```python
from build123d import *

# Parameters (mm, degrees)
SKETCH1_R                = 1.8
BOSS_EXTRUDE1_DEPTH      = 2
BOSS_EXTRUDE2_DEPTH      = 33
BOSS_EXTRUDE3_DEPTH      = 1
CHAMFER1_START           = 78.15897378
CHAMFER1_DEPTH           = 1.443375673
BOSS_EXTRUDE4_DEPTH      = 3
BOSS_EXTRUDE4_DEPTH_BACK = 0.0001
BOSS_EXTRUDE5_DEPTH      = 2.5
CUT_EXTRUDE1_DEPTH       = 3.0001


with BuildPart() as part:
    # Sketch1 → Boss-Extrude1 (new body)
    with BuildSketch(Plane(origin=(34.895003496, 0, 0), x_dir=(0, 0, -1), z_dir=(1, 0, 0))):
        with BuildLine():
            Line((-197.649446246, 296.929756404), (-189.949446246, 296.929756404))
            Line((-189.949446246, 296.929756404), (-189.949446246, 254.929756404))
            Line((-189.949446246, 254.929756404), (-196.543558796, 254.929756404))
            Line((-196.543558796, 254.929756404), (-231.255333696, 254.929756404))
            Line((-231.255333696, 254.929756404), (-234.649446246, 258.323868954))
            Line((-234.649446246, 258.323868954), (-234.649446246, 304.785643855))
            Line((-234.649446246, 304.785643855), (-231.255333696, 308.179756404))
            Line((-231.255333696, 308.179756404), (-227.755333696, 308.179756404))
            Line((-227.755333696, 308.179756404), (-224.361221147, 304.785643855))
            Line((-224.361221147, 304.785643855), (-220.634013353, 301.058436061))
            ThreePointArc((-220.634013353, 301.058436061), (-219.660743306, 300.408117807), (-218.512693009, 300.179756404))
            Line((-218.512693009, 300.179756404), (-213.899446246, 300.179756404))
            ThreePointArc((-213.899446246, 300.179756404), (-211.430377525, 299.74636844), (-209.256499056, 298.498018377))
            Line((-209.256499056, 298.498018377), (-208.488462922, 297.857611868))
            ThreePointArc((-208.488462922, 297.857611868), (-207.289081698, 297.168867005), (-205.926836886, 296.929756404))
            Line((-205.926836886, 296.929756404), (-197.649446246, 296.929756404))
        make_face()
        with Locations(Location((-198.399446246, 291.179756404, 0), (0, 0, 90))):
            Circle(SKETCH1_R, mode=Mode.SUBTRACT)
        with Locations(Location((-198.399446246, 260.179756404, 0), (0, 0, 90))):
            Circle(SKETCH1_R, mode=Mode.SUBTRACT)
        with Locations(Location((-229.399446246, 260.179756404, 0), (0, 0, 90))):
            Circle(SKETCH1_R, mode=Mode.SUBTRACT)
    extrude(amount=BOSS_EXTRUDE1_DEPTH)

    # Sketch2 → Boss-Extrude2 (add)
    with BuildSketch(Plane.ZY.offset(-34.895003496)):
        Polygon((192.949446246, 296.929756404), (192.949446246, 255.737509851), (192.949446246, 254.929756404), (189.949446246, 254.929756404), (189.949446246, 296.929756404), align=None)
    extrude(amount=BOSS_EXTRUDE2_DEPTH)

    # Sketch3 → Boss-Extrude3 (add)
    with BuildSketch(Plane(origin=(0, 296.929756404, 0), x_dir=(1, 0, 0), z_dir=(0, 1, 0))):
        Polygon((24.09465277, -192.949446246), (34.895003496, -196.599446246), (34.895003496, -192.949446246), align=None)
    extrude(amount=-BOSS_EXTRUDE3_DEPTH)

    # Chamfer1: read off the stored shape, not the designer's step
    # Chamfer1 outline → Chamfer1 (add)
    with BuildSketch(Plane(origin=(0, 0, 0), x_dir=(0.8164965809277265, -0.4082482904638619, 0.4082482904638633), z_dir=(0.5773502691896251, 0.5773502691896252, -0.5773502691896272)).offset(CHAMFER1_START)):
        Polygon((-15.59112598, -345.689799375), (-12.529263801, -347.457566328), (-12.529263801, -343.922032422), align=None)
    extrude(amount=CHAMFER1_DEPTH)

    # Sketch4 → Boss-Extrude4 (add, two sides: drawn at the far end of the back side and taken through both)
    with BuildSketch(Plane.XZ.offset(-254.929756404).offset(-BOSS_EXTRUDE4_DEPTH_BACK)):
        Polygon((1.895003496, 192.949446246), (34.895003496, 192.949446246), (34.895003496, 231.255333696), (36.895003496, 231.255333696), (36.895003496, 189.949446246), (1.895003496, 170.0501531), align=None)
    extrude(amount=BOSS_EXTRUDE4_DEPTH + BOSS_EXTRUDE4_DEPTH_BACK)

    # Sketch5 → Boss-Extrude5 (add)
    with BuildSketch(Plane.XZ.offset(-251.929756404)):
        Polygon((11.795887964, 192.949446246), (34.895003496, 212.102389971), (34.895003496, 192.949446246), align=None)
    extrude(amount=-BOSS_EXTRUDE5_DEPTH)

    # Sketch6 → Cut-Extrude1 (cut)
    with BuildSketch(Plane(origin=(0, 254.929856404, 0), x_dir=(1, 0, 0), z_dir=(0, 1, 0))):
        Polygon((1.895003496, -189.949446246), (36.895003496, -189.949446246), (1.895003496, -170.0501531), align=None)
    extrude(amount=-CUT_EXTRUDE1_DEPTH, mode=Mode.SUBTRACT)


solid = part.part
```
The model under review builds one solid part; all positions refer to its coordinate system, in mm. A direction names the side the tool comes from. Round coordinates to 2 decimals unless told otherwise and drop trailing zeros. Loops run counter-clockwise (first coordinate to the right, second up) from the corner with the lowest first, then second, coordinate; pieces in that order, holes last. Notation, with made-up numbers: (56.5, 65) - (78.5, 65) arc R16 ccw to (78.5, 77) - close; hole circle Ø3 at (73.25, 47). An arc over 180 degrees is marked (long way). Use a Markdown table: item, result. Add a question column.
Q1. Add section B-B (x = 33.5). State the section outline as (y, z) points.
Q2. Add section D-D (y = 288). State the section outline as (x, z) points (3 decimals), plus the area to 3 significant figures.
Q3. Add section C-C (z = 199.5). State the section outline as (x, y) points (3 decimals), plus the area to 3 significant figures.
Q4. For probe 1 along Z at (x, y) = (32, 257.5); probe 2 along X at (y, z) = (261, 225.5) (3 decimals); probe 3 along Y at (x, z) = (28, 195.5), list the stretches that pass through material, from the lowest coordinate up.
Q5. Insertion check: pin 1 Ø16.5 at (x, y) = (18.5, 280.5) entering from +Z; pin 2 Ø8 at (x, z) = (17, 198.5) entering from +Y; pin 3 Ø2 at (y, z) = (260.18, 229.4) entering from +X; pin 4 Ø10 at (x, z) = (31.5, 219) entering from +Y. Each pin has a flat end and moves straight along its axis. Give the tip position at first contact, or say it passes through.
Q6. Add section A-A (z = 230.5). State the section outline as (x, y) points (3 decimals).
Q7. Machinability: for faces 4 (the face through (18, 275, 192.949)), 5 (the face through (35.881, 258.853, 230.616)), 6 (the face through (29.42, 296.44, 194.75)), which of the approach directions +Z, -Z, +X, -X, +Y, -Y give a long, thin tool a straight path to every point of the face, cutting with its end or side? Answer none if there is none.
Q8. The part is to be moulded in two halves that separate along Z. For faces 1 (the face through (23, 296.93, 192)), 2 (the face through (35.881, 258.853, 199.616)), 3 (the face through (36, 253, 231.255)), say which applies: pulls with the +Z half, pulls with the -Z half, needs draft (parallel to the pull), parting line crosses it, or undercut.
Worked answers:
| question | item | result |
|---|---|---|
| 1 | outline | (251.93, 189.95) - (296.93, 189.95) - (296.93, 196.13) - (295.93, 196.13) - (295.93, 194.05) - (294.82, 192.95) - (254.43, 192.95) - (254.43, 210.95) - (251.93, 210.95) - close |
| 2 | outline | (1.895, 189.949) - (36.895, 189.949) - (36.895, 234.649) - (34.895, 234.649) - (34.895, 192.949) - (1.895, 192.949) - close |
| 2 | area | 188 mm² |
| 3 | outline | (19.696, 251.93) - (36.895, 251.93) - (36.895, 258.755) - (34.895, 258.755) - (34.895, 254.43) - (19.696, 254.43) - close; (34.895, 261.604) - (36.895, 261.604) - (36.895, 289.755) - (34.895, 289.755) - close; (34.895, 292.604) - (36.895, 292.604) - (36.895, 296.93) - (34.895, 296.93) - close |
| 3 | area | 117 mm² |
| 4 | probe 1 | 189.95 to 192.95 |
| 4 | probe 2 | 34.895 to 36.895 |
| 4 | probe 3 | 251.93 to 254.43 |
| 5 | pin 1 | z = 192.95 |
| 5 | pin 2 | y = 254.43 |
| 5 | pin 3 | through |
| 5 | pin 4 | y = 303.1 |
| 6 | outline | (34.895, 251.93) - (36.895, 251.93) - (36.895, 258.755) - (34.895, 258.755) - close; (34.895, 261.604) - (36.895, 261.604) - (36.895, 308.18) - (34.895, 308.18) - close |
| 7 | face 4 | +Z, -X |
| 7 | face 5 | +X, -X |
| 7 | face 6 | +Z, -X, +Y |
| 8 | face 1 | needs draft |
| 8 | face 2 | undercut |
| 8 | face 3 | pulls with the +Z half |
